```python
from build123d import *

# Parameters (mm, degrees)
F1_DEPTH = 16


with BuildPart() as f1:
    # F0 (on Front) → F1 (new body)
    with BuildSketch(Plane.XZ):
        with BuildLine():
            Line((95.341194, 8.899506), (1.341194, 8.899506))
            ThreePointArc((1.341194, 8.899506), (-8.974841, 0.672477), (0, -9))
            Line((0, -9), (19, -9))
            ThreePointArc((19, -9), (20.604423, -9.264409), (22.039157, -10.02967))
            ThreePointArc((22.039157, -10.02967), (70.763703, -36.139738), (125.254312, -45.445144))
            ThreePointArc((125.254312, -45.445144), (129.154135, -46.415554), (132.617611, -48.45385))
            Line((132.617611, -48.45385), (134.065223, -46.76863))
            ThreePointArc((134.065223, -46.76863), (128.853194, -44.058853), (123.014468, -43.412776))
            ThreePointArc((123.014468, -43.412776), (70.347282, -33.878442), (23.25482, -8.441537))
            ThreePointArc((23.25482, -8.441537), (21.246192, -7.370172), (19, -7))
            Line((19, -7), (0, -7))
            ThreePointArc((0, -7), (-6.974831, 0.593069), (1.181873, 6.899506))
            Line((1.181873, 6.899506), (95.181873, 6.899506))
            Line((95.181873, 6.899506), (95.341194, 8.899506))
        make_face()
    extrude(amount=F1_DEPTH)


solid = f1.part
```
Input: part model. Units: mm. Frame: model coordinates. A direction names the side the tool comes from. Give positions to 0.01 mm unless a question says otherwise; leave off trailing zeros. Order: outer loops, then holes, each group sorted by start corner. A loop starts at its lowest first (then second) coordinate and runs counter-clockwise, first axis right, second up.
1. Section C-C on z = 0. Return the cut outline in (x, y), and give its area (3 significant figures).
Derived:
outline: (-9, -16) - (-7, -16) - (-7, 0) - (-9, 0) - close
area: 32.0 mm2
2. Pin query (flat end, axial travel): pin 1 (5 mm diameter, centred on x = 26.5, y = -12.5, fed in from -Z); pin 2 (2 mm diameter, centred on x = 33, y = -7.5, fed in from -Z); pin 3 (5 mm diameter, centred on x = 73.5, y = -8, fed in from -Z); pin 4 (5 mm diameter, centred on x = 50.5, z = -22.5, fed in from +Y). Return the tip coordinate at first contact, or that it passes through.
Derived:
pin 1: stops at z = -15.09
pin 2: stops at z = -18.4
pin 3: stops at z = -37.84
pin 4: passes through
3. Reachability of faces 1 (the flat face through (46, 0, -24)), 2 (the cylindrical face through (21.28, -7.89, -7.38)), 3 (the flat face through (49, -8, 8.9)), 4 (the flat face through (9, -8, -9)), 5 (the flat face through (46, -16, -24)) from +Z, -Z, +X, -X, +Y, -Y: full face, straight path, thin tool, end or side. Return the list, or none.
Derived:
face 1: +Z, -Z, +X, -X, +Y
face 2: +X, +Y, -Y
face 3: +Z, +X, +Y, -Y
face 4: -Z, -X, +Y, -Y
face 5: +Z, -Z, +X, -X, -Y
4. Section D-D on x = 116. Return the cut outline in (y, z), and give its area (3 significant figures).
Derived:
outline: (-16, -45.12) - (0, -45.12) - (0, -43.12) - (-16, -43.12) - close
area: 32.1 mm2
5. Material intervals for L1, parallel to Z at x = 0, y = -9; L2, parallel to X at y = -5, z = 0; L3, parallel to Z at x = 26, y = -10, sorted ascending.
Derived:
L1: z = -9 to -7, 7 to 9
L2: x = -9 to -7
L3: z = -12.97 to -10.5, 6.9 to 8.9
6. Mould query, pull axis Z, two halves, no side actions, for faces 6 (the cylindrical face through (128.932, -7.888, -44.083)), 7 (the cylindrical face through (70.029, -7.888, -35.886)), 8 (the flat face through (48, -8, 6.9)), 9 (the cylindrical face through (-8.957, -7.888, 0.879)). Classes: released by +Z, released by -Z, zero draft, split by the parting line, or undercut.
Derived:
face 6: released by +Z
face 7: released by -Z
face 8: undercut
face 9: split by the parting line
7. Section B-B on y = -5.75. Return the cut outline in (x, z), and give its area (3 significant figures).
Derived:
outline: (0, -9) - (19, -9) arc R5 cw to (22.04, -10.03) arc R172 ccw to (125.25, -45.45) arc R14 cw to (132.62, -48.45) - (134.07, -46.77) arc R16 ccw to (123.01, -43.41) arc R170 cw to (23.25, -8.44) arc R7 ccw to (19, -7) - (0, -7) arc R7 cw (long way) to (1.18, 6.9) - (95.18, 6.9) - (95.34, 8.9) - (1.34, 8.9) arc R9 ccw (long way) to start
area: 526 mm2
8. Section A-A on x = 68. Return the cut outline in (y, z).
Derived:
outline: (-16, -35.17) - (0, -35.17) - (0, -33.04) - (-16, -33.04) - close; (-16, 6.9) - (0, 6.9) - (0, 8.9) - (-16, 8.9) - close
